Could you check a few things on this model? Use its own coordinates, in mm. Round coordinates to 2 decimals unless told otherwise and drop trailing zeros. Order: outer loops, then holes, each group sorted by start corner. A loop starts at its lowest first (then second) coordinate and runs counter-clockwise, first axis right, second up. Notation, with made-up numbers: (87.5, 51.5) - (115.5, 51.5) arc R32 ccw to (115.5, 83.5) - close; hole circle Ø5 at (19.25, 37.25). An arc over 180 degrees is marked (long way). Return JSON: item names as keys, results as strings. Group by question number.
Autodesk Inventor part; units mm, degrees
ref_plane "YZ Plane" through (0, 0, 0) normal (1, 0, 0) x (0, 1, 0)
ref_plane "XZ Plane" through (0, 0, 0) normal (0, 1, 0) x (-1, 0, 0)
ref_plane "XY Plane" through (0, 0, 0) normal (0, 0, 1) x (1, 0, 0)
sketch "Sketch1" plane through (0, 0, 0) normal (0, 1, 0) x (-1, 0, 0)
  line L0 (0, 0) -> (38.1, 0)
  line L1 (38.1, 0) -> (38.1, -93.98)
  line L2 (38.1, -93.98) -> (0, -93.98)
  line L3 (0, -93.98) -> (0, 0)
  dimension "d0" = 38.1
  dimension "d1" = 93.98
extrude "Extrusion1" add sketch "Sketch1" along normal blind 1.778
fillet "Fillet1" radius 1.27 4 edges at (0, 0.889, 0) (0, 0.889, -93.98) (-38.1, 0.889, -93.98) (-38.1, 0.889, 0)
sketch "Sketch3" plane through (0, 1.778, 0) normal (0, 1, 0) x (1, 0, 0)
  arc A0 (-38.1, 1.27) -> (-36.83, 0) centre (-36.83, 1.27) ccw
  line L0 (-36.83, 0) -> (-1.27, 0)
  arc A1 (-1.27, 0) -> (0, 1.27) centre (-1.27, 1.27) ccw
  line L1 (0, 1.27) -> (0, 92.71)
  arc A2 (0, 92.71) -> (-1.27, 93.98) centre (-1.27, 92.71) ccw
  line L2 (-1.27, 93.98) -> (-36.83, 93.98)
  arc A3 (-36.83, 93.98) -> (-38.1, 92.71) centre (-36.83, 92.71) ccw
  line L3 (-38.1, 92.71) -> (-38.1, 1.27)
  line L4 (-35.814, 2.286) -> (-2.286, 2.286)
  line L5 (-2.286, 4.826) -> (-2.286, 89.154)
  line L6 (-2.286, 91.694) -> (-35.814, 91.694)
  line L7 (-35.814, 89.154) -> (-35.814, 4.826)
  line L8 (-34.29, 3.302) -> (-3.81, 3.302)
  line L9 (-34.29, 90.678) -> (-3.81, 90.678)
  arc A4 (-35.814, 4.826) -> (-34.29, 3.302) centre (-34.29, 4.826) ccw
  arc A5 (-3.81, 3.302) -> (-2.286, 4.826) centre (-3.81, 4.826) ccw
  arc A6 (-2.286, 89.154) -> (-3.81, 90.678) centre (-3.81, 89.154) ccw
  arc A7 (-34.29, 90.678) -> (-35.814, 89.154) centre (-34.29, 89.154) ccw
  point P0 (0, 0)
  dimension "d9" = 2.286
  dimension "d10" = 1.016
  dimension "d11" = 1.016
  dimension "d12" = 1.524
extrude "Extrusion3" cut sketch "Sketch3" against normal through all contours A5 L8 A4 L7 A7 L9 A6 L5
properties part number "TopCoverContactSpacer" material "ABS Plastic"
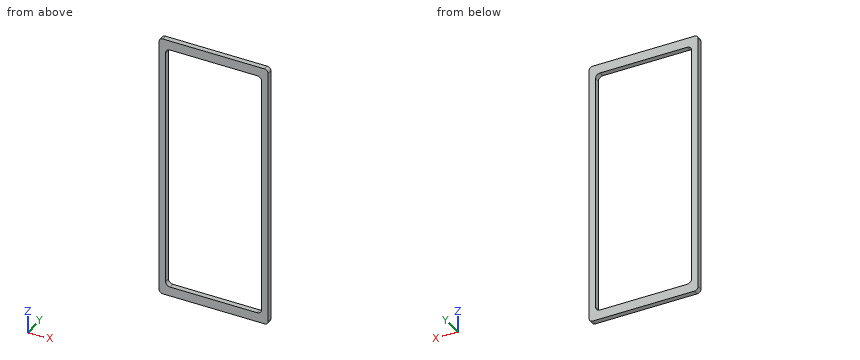
1) I want a section at B-B, the plane y = 0.95. List the corners of the cut face in (x, z) for me, plus the area to 3 significant figures.
2) I want a section at A-A, the plane z = -74.5. List the corners of the cut face in (x, y) for me, plus the area to 3 significant figures.
3) I want a section at C-C, the plane x = -27. List the corners of the cut face in (y, z) for me, plus the area to 3 significant figures.
4) Will this pin go through, and if not, where does the flat tip stop? pin 1 (4 mm diameter, centred on x = -5, z = -39, fed in from +Y).
5) If I drill on line 1 along X through (y, z) = (0.9, -43); line 2 along Z through (x, y) = (-26, 0.55); line 3 along Z through (x, y) = (-37, 0.1), over which ranges is the centre line in solid material (lowest first)? Write a range as from..to.
Outcome:
{
 "1": {"outline": "(-38.1, -92.71) arc R1.27 ccw to (-36.83, -93.98) - (-1.27, -93.98) arc R1.27 ccw to (0, -92.71) - (0, -1.27) arc R1.27 ccw to (-1.27, 0) - (-36.83, 0) arc R1.27 ccw to (-38.1, -1.27) - close; hole (-35.81, -89.15) arc R1.52 ccw to (-34.29, -90.68) - (-3.81, -90.68) arc R1.52 ccw to (-2.29, -89.15) - (-2.29, -4.83) arc R1.52 ccw to (-3.81, -3.3) - (-34.29, -3.3) arc R1.52 ccw to (-35.81, -4.83) - close", "area": "652 mm^2"},
 "2": {"outline": "(-38.1, 0) - (-35.81, 0) - (-35.81, 1.78) - (-38.1, 1.78) - close; (-2.29, 0) - (0, 0) - (0, 1.78) - (-2.29, 1.78) - close", "area": "8.13 mm^2"},
 "3": {"outline": "(0, -93.98) - (1.78, -93.98) - (1.78, -90.68) - (0, -90.68) - close; (0, -3.3) - (1.78, -3.3) - (1.78, 0) - (0, 0) - close", "area": "11.7 mm^2"},
 "4": {"pin 1": "through"},
 "5": {"line 1": "-38.1..-35.81, -2.29..0", "line 2": "-93.98..-90.68, -3.3..0", "line 3": "-93.97..-0.01"}
}
